from build123d import *

# Parameters (mm, degrees)
SKETCH126_W  = 5.7
SKETCH126_H  = 3.8
PAD061_DEPTH = 1.7
SKETCH127_W  = 6.5
SKETCH127_H  = 5.205
PAD062_DEPTH = 1.6
SKETCH128_W  = 6.5
SKETCH128_H  = 6.205
PAD063_DEPTH = 2
CHAMFER_SIZE = 1


with BuildPart() as part:
    # Sketch126 → Pad061 (new body)
    with BuildSketch(Plane.YZ):
        with Locations((-7.89, 11.095)):
            Rectangle(SKETCH126_W, SKETCH126_H)
    extrude(amount=PAD061_DEPTH)

    # Sketch127 → Pad062 (join)
    with BuildSketch(Plane.YZ.offset(1.7)):
        with Locations((-7.89, 10.3925)):
            Rectangle(SKETCH127_W, SKETCH127_H)
    extrude(amount=PAD062_DEPTH)

    # Sketch128 → Pad063 (join)
    with BuildSketch(Plane.YZ):
        with Locations((-7.89, 9.8925)):
            Rectangle(SKETCH128_W, SKETCH128_H)
    extrude(amount=-PAD063_DEPTH)

    # Chamfer
    chamfer_edges = [part.edges().sort_by_distance(p)[0] for p in [
        (-2, -7.89, 12.995),
        (-2, -11.14, 9.8925),
        (-2, -7.89, 6.79),
        (-2, -4.64, 9.8925),
    ]]
    chamfer(chamfer_edges, length=CHAMFER_SIZE)


with BuildPart() as part_1:
    # Body017 placement: moved
    add(part.part.moved(Location((-29.5, 0, 0))))


solid = part_1.part
Check sheet for the modelled part. Datum: model origin and axes. Units: mm. A direction names the side the tool comes from. Round coordinates to 2 decimals unless told otherwise and drop trailing zeros. Write each loop counter-clockwise with the first axis right and the second up, starting at its lowest first coordinate (ties: lowest second). Pieces come first, ordered by that corner, then holes. Notation, with made-up numbers: (34, 73.25) - (91, 73.25) arc R11 cw to (91, 87.25) - close; hole circle Ø6 at (30.25, 35.25). An arc over 180 degrees is marked (long way). Return JSON: item names as keys, results as strings.
Q1. Cross-section at B-B (y = -6.75). Record the boundary of the cut face in (x, z) (3 decimals), then the cut area to 3 significant figures.
Returned:
{"outline": "(-31.5, 7.79) - (-30.5, 6.79) - (-29.5, 6.79) - (-29.5, 9.195) - (-27.8, 9.195) - (-27.8, 7.79) - (-26.2, 7.79) - (-26.2, 12.995) - (-30.5, 12.995) - (-31.5, 11.995) - close", "area": "26.2 mm²"}
Q2. Scan lines: L1, parallel to X at y = -6, z = 9; L2, parallel to Z at x = -28.65, y = -6.75 (3 decimals); L3, parallel to Y at x = -28.25, z = 10.5. Record each from-to range of solid material in increasing order. Write a range as from..to.
Returned:
{"L1": "x = -31.5..-29.5, -27.8..-26.2", "L2": "z = 9.195..12.995", "L3": "y = -10.74..-5.04"}
Q3. Cross-section at C-C (z = 9.5). Record the boundary of the cut face in (x, y).
Returned:
{"outline": "(-31.5, -10.14) - (-30.5, -11.14) - (-29.5, -11.14) - (-29.5, -10.74) - (-27.8, -10.74) - (-27.8, -11.14) - (-26.2, -11.14) - (-26.2, -4.64) - (-27.8, -4.64) - (-27.8, -5.04) - (-29.5, -5.04) - (-29.5, -4.64) - (-30.5, -4.64) - (-31.5, -5.64) - close"}
Q4. Cross-section at D-D (x = -27.05). Record the boundary of the cut face in (y, z) (3 decimals).
Returned:
{"outline": "(-11.14, 7.79) - (-4.64, 7.79) - (-4.64, 12.995) - (-11.14, 12.995) - close"}
Q5. Depth check by flat-ended pin: P1, Ø0.8, axis at x = -29, z = 10.5, coming from the -Y side; P2, Ø1.5, axis at x = -27.5, y = -7.5, coming from the -Z side; P3, Ø0.8, axis at x = -28.5, z = 11, coming from the +Y side. Enter the tip coordinate at first touch or a pass-through.
Returned:
{"P1": "stops at y = -10.74", "P2": "stops at z = 7.79", "P3": "stops at y = -5.04"}
Q6. Access from +Z, -Z, +X, -X, +Y, -Y to the whole of each face (thin tool, end or side, straight path). Record for faces 1 (the flat face through (-29, -8, 9.195)), 2 (the flat face through (-29, -5.04, 11)), 3 (the flat face through (-29, -10.74, 11)).
Returned:
{"face 1": "-Z, +Y, -Y", "face 2": "+Z, -Z, +Y", "face 3": "+Z, -Z, -Y"}
Q7. Cross-section at A-A (z = 8.5). Record the boundary of the cut face in (x, y).
Returned:
{"outline": "(-31.5, -10.14) - (-30.5, -11.14) - (-29.5, -11.14) - (-29.5, -4.64) - (-30.5, -4.64) - (-31.5, -5.64) - close; (-27.8, -11.14) - (-26.2, -11.14) - (-26.2, -4.64) - (-27.8, -4.64) - close"}
Q8. Draft check along X on faces 4 (the flat face through (-30, -4.64, 10)), 5 (the flat face through (-29.5, -9, 9)), 6 (the flat face through (-31.01, -7.94, 7.3)), 7 (the flat face through (-26.2, -8, 10)). Enter one of: released by +X, released by -X, zero draft, split by the parting line, or undercut.
Returned:
{"face 4": "zero draft", "face 5": "undercut", "face 6": "released by -X", "face 7": "released by +X"}
